Verification items for the finished model (mm, model axes). A direction names the side the tool comes from. Give positions to 0.01 mm unless a question says otherwise; leave off trailing zeros. Write each loop counter-clockwise with the first axis right and the second up, starting at its lowest first coordinate (ties: lowest second). Pieces come first, ordered by that corner, then holes. Notation, with made-up numbers: (67.25, 47) -> (90.25, 47) arc R26 cw to (90.25, 65) -> close; hole circle Ø4 at (6, -18.5). An arc over 180 degrees is marked (long way). Write item = value, one per line.
from build123d import *

# Parameters (mm, degrees)
EXTRUDE_1_DEPTH     = 30
SKETCH_2_R          = 3
CUT_EXTRUDE_1_DEPTH = 22
CUT_EXTRUDE_2_DEPTH = 30


with BuildPart() as part:
    # 스케치1 → 보스-돌출1 (new body)
    with BuildSketch(Plane.XY):
        with BuildLine():
            Line((40, 11), (65, 11))
            Line((65, 11), (65, -11))
            Line((65, -11), (40, -11))
            ThreePointArc((40, -11), (39.853553391, -10.646446609), (39.5, -10.5))
            Line((39.5, -10.5), (-39.5, -10.5))
            ThreePointArc((-39.5, -10.5), (-39.853553391, -10.646446609), (-40, -11))
            Line((-40, -11), (-65, -11))
            Line((-65, -11), (-65, 11))
            Line((-65, 11), (-40, 11))
            ThreePointArc((-40, 11), (-39.853553391, 10.646446609), (-39.5, 10.5))
            Line((-39.5, 10.5), (39.5, 10.5))
            ThreePointArc((39.5, 10.5), (39.853553391, 10.646446609), (40, 11))
        make_face()
    extrude(amount=EXTRUDE_1_DEPTH)

    # 스케치2 → 컷-돌출1 (cut)
    with BuildSketch(Plane(origin=(0, 11, 0), x_dir=(1, 0, 0), z_dir=(0, 1, 0))):
        with Locations((52.5, -7.5)):
            Circle(SKETCH_2_R)
        with Locations((52.5, -22.5)):
            Circle(SKETCH_2_R)
        with Locations((-52.5, -7.5)):
            Circle(SKETCH_2_R)
        with Locations((-52.5, -22.5)):
            Circle(SKETCH_2_R)
    extrude(amount=-CUT_EXTRUDE_1_DEPTH, mode=Mode.SUBTRACT)

    # 스케치4 → 컷-돌출2 (cut)
    with BuildSketch(Plane(origin=(0, 0, 0), x_dir=(-1, 0, 0), z_dir=(0, 0, -1))):
        with BuildLine():
            Line((-18.222279144, 4.25), (18.222279144, 4.25))
            ThreePointArc((18.222279144, 4.25), (33, 0), (18.222279144, -4.25))
            Line((18.222279144, -4.25), (-18.222279144, -4.25))
            ThreePointArc((-18.222279144, -4.25), (-33, 0), (-18.222279144, 4.25))
        make_face()
    extrude(amount=-CUT_EXTRUDE_2_DEPTH, mode=Mode.SUBTRACT)


solid = part.part
Item 1: Mould release check, pull along Z, two halves, no side actions. Record for faces 1 (the cylindrical face through (33, 0, 15)), 2 (the flat face through (1, 5, 0)), 3 (the flat face through (1, 5, 30)), 4 (the cylindrical face through (-55.5, 0.2, 22.4)): +Z half, -Z half, draft (parallel to the pull), parting line (faces both ways), or undercut.
Response values:
face_1 = draft
face_2 = -Z half
face_3 = +Z half
face_4 = undercut
Item 2: Material ranges on line 1 (Z direction, x = 52.5, y = 5); line 2 (Y direction, x = 25, z = 16); line 3 (X direction, y = 1, z = 22.5), recorded low to high.
Response values:
line_1 = 0 to 4.5, 10.5 to 19.5, 25.5 to 30
line_2 = -10.5 to -8, 8 to 10.5
line_3 = -65 to -55.5, -49.5 to -32.94, 32.94 to 49.5, 55.5 to 65
Item 3: Sectioned sample at A-A on x = 52.5. Record the cut outline in (y, z), then the cut area to 3 significant figures.
Response values:
outline = (-11, 0) -> (11, 0) -> (11, 4.5) -> (-11, 4.5) -> close; (-11, 10.5) -> (11, 10.5) -> (11, 19.5) -> (-11, 19.5) -> close; (-11, 25.5) -> (11, 25.5) -> (11, 30) -> (-11, 30) -> close
area = 396 mm^2
Item 4: Go/stop test with flat-tipped pins: P1, Ø7, axis at x = 52.5, z = 22.5, coming from the -Y side; P2, Ø9, axis at x = 5, z = 11, coming from the +Y side; P3, Ø9, axis at x = 19.5, z = 18.5, coming from the -Y side. Record where each tip stops, or that it passes through.
Response values:
P1 = -11
P2 = 10.5
P3 = -10.5
Item 5: Sectioned sample at B-B on z = 22.5. Record the cut outline in (x, y), then the cut area to 3 significant figures.
Response values:
outline = (-65, -11) -> (-55.5, -11) -> (-55.5, 11) -> (-65, 11) -> close; (-49.5, -11) -> (-40, -11) arc R0.5 cw to (-39.5, -10.5) -> (39.5, -10.5) arc R0.5 cw to (40, -11) -> (49.5, -11) -> (49.5, 11) -> (40, 11) arc R0.5 cw to (39.5, 10.5) -> (-39.5, 10.5) arc R0.5 cw to (-40, 11) -> (-49.5, 11) -> close; (55.5, -11) -> (65, -11) -> (65, 11) -> (55.5, 11) -> close; hole (-18.22, -4.25) -> (18.22, -4.25) arc R8 ccw (long way) to (18.22, 4.25) -> (-18.22, 4.25) arc R8 ccw (long way) to start
area = 1,820 mm^2
Item 6: Set-up check for faces 5 (the flat face through (0, 4.25, 15)), 6 (the flat face through (65, 0, 15)), 7 (the flat face through (53, -11, 15)), 8 (the flat face through (1, -10.5, 15)), 9 (the flat face through (-1, 10.5, 15)): record each of +Z, -Z, +X, -X, +Y, -Y from which the full face is reachable in a straight line by a thin tool's end or side.
Response values:
face_5 = +Z, -Z
face_6 = +Z, -Z, +X, +Y, -Y
face_7 = +Z, -Z, +X, -X, -Y
face_8 = +Z, -Z, -Y
face_9 = +Z, -Z, +Y
Item 7: Sectioned sample at D-D on z = 14.25. Record the cut outline in (x, y), then the cut area to 3 significant figures.
Response values:
outline = (-65, -11) -> (-40, -11) arc R0.5 cw to (-39.5, -10.5) -> (39.5, -10.5) arc R0.5 cw to (40, -11) -> (65, -11) -> (65, 11) -> (40, 11) arc R0.5 cw to (39.5, 10.5) -> (-39.5, 10.5) arc R0.5 cw to (-40, 11) -> (-65, 11) -> close; hole (-18.22, -4.25) -> (18.22, -4.25) arc R8 ccw (long way) to (18.22, 4.25) -> (-18.22, 4.25) arc R8 ccw (long way) to start
area = 2,080 mm^2
Item 8: Sectioned sample at C-C on y = 6.5. Record the cut outline in (x, z), then the cut area to 3 significant figures.
Response values:
outline = (-65, 0) -> (-29.66, 0) -> (-29.66, 30) -> (-65, 30) -> close; (-20.34, 0) -> (20.34, 0) -> (20.34, 30) -> (-20.34, 30) -> close; (29.66, 0) -> (65, 0) -> (65, 30) -> (29.66, 30) -> close; hole circle Ø6 at (-52.5, 7.5); hole circle Ø6 at (-52.5, 22.5); hole circle Ø6 at (52.5, 7.5); hole circle Ø6 at (52.5, 22.5)
area = 3,230 mm^2
